Geometry: final body of the model. Coordinates: model frame, mm. Face numbers are marked on the shaded views. A direction names the side the tool comes from. Give positions to 0.01 mm unless a question says otherwise; leave off trailing zeros. Write each loop counter-clockwise with the first axis right and the second up, starting at its lowest first coordinate (ties: lowest second). Pieces come first, ordered by that corner, then holes. Notation, with made-up numbers: M -10.5,57.25 L 18.5,57.25 A26 ccw 18.5,80.25 Z; hole C 51.5,-28 d1. An arc over 180 degrees is marked long. One line per question, with ' | ' between items.
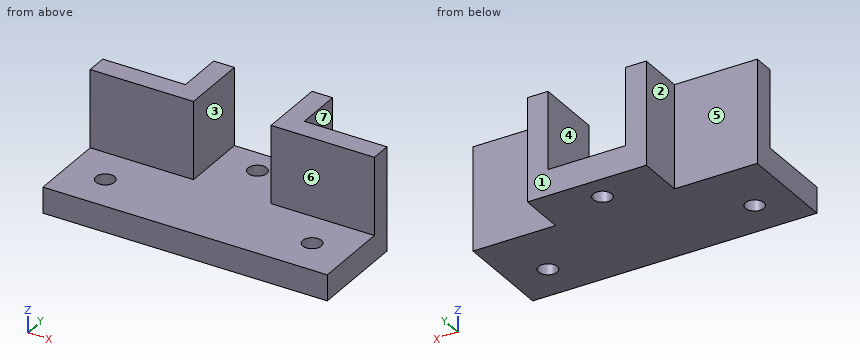
from build123d import *

# Parameters (mm, degrees)
BOSS_EXTRUDE1_DEPTH = 5
BOSS_EXTRUDE2_DEPTH = 20
SKETCH6_R           = 1.8
CUT_EXTRUDE3_DEPTH  = 6


with BuildPart() as part:
    # Sketch1 → Boss-Extrude1 (new body)
    with BuildSketch(Plane.XY):
        Polygon((14.31372549, 2.735294118), (34.31372549, 2.735294118), (34.31372549, -12.264705882), (-20.68627451, -12.264705882), (-20.68627451, 2.735294118), (-0.68627451, 2.735294118), (-0.68627451, 15.735294118), (14.31372549, 15.735294118), align=None)
    extrude(amount=BOSS_EXTRUDE1_DEPTH)

    # Sketch2 → Boss-Extrude2 (add)
    with BuildSketch(Plane(origin=(0, 0, 0), x_dir=(-1, 0, 0), z_dir=(0, 0, -1))):
        Polygon((0.68627451, 15.735294118), (4.68627451, 15.735294118), (4.68627451, 6.735294118), (6.079970528, 6.735294118), (20.68627451, 6.735294118), (20.68627451, 2.735294118), (0.68627451, 2.735294118), align=None)
    boss_extrude2 = extrude(amount=-BOSS_EXTRUDE2_DEPTH)

    # Mirror1: Boss-Extrude2 across plane
    add(boss_extrude2.mirror(Plane.ZY.offset(-6.81372549)))

    # Sketch6 → Cut-Extrude3 (cut, through all)
    with BuildSketch(Plane.XY.offset(5)):
        with Locations((6.81372549, 10.735294118)):
            Circle(SKETCH6_R)
        with Locations((-13.18627451, -4.764705882)):
            Circle(SKETCH6_R)
        with Locations((26.81372549, -4.764705882)):
            Circle(SKETCH6_R)
    extrude(amount=-CUT_EXTRUDE3_DEPTH, mode=Mode.SUBTRACT)


solid = part.part
(1) Cut plane A-A, the plane z = 6.75. Return loops of the section in (x, y).
Working result:
outline: M -20.69,2.74 L -0.69,2.74 L -0.69,15.74 L -4.69,15.74 L -4.69,6.74 L -20.69,6.74 Z; M 14.31,2.74 L 34.31,2.74 L 34.31,6.74 L 18.31,6.74 L 18.31,15.74 L 14.31,15.74 Z
(2) Material intervals for L1, parallel to X at y = 5, z = 14.5; L2, parallel to X at y = 14, z = 11.5; L3, parallel to X at y = -5, z = 1.75, sorted ascending. Write a range as [from, to].
Working result:
L1: x = [-20.69, -0.69], [14.31, 34.31] | L2: x = [-4.69, -0.69], [14.31, 18.31] | L3: x = [-20.69, -14.97], [-11.4, 25.03], [28.6, 34.31]
(3) Set-up query: the marked faces 4, 5, 6 and 7. Return all of +Z, -Z, +X, -X, +Y, -Y with unobstructed straight access to the full face (end or side cutting, diameter ignored); none if empty.
Working result:
face 4: +Z, +Y, -Y | face 5: +Z, -Z, -X, +Y | face 6: +Z, +X, -X, -Y | face 7: +Z, -Z, +X, +Y
(4) First-contact query: P1, Ø12, axis at x = 28, z = 11.5, coming from the -Y side; P2, Ø4, axis at x = 3.5, y = -6, coming from the +Z side; P3, Ø4.5, axis at y = 13, z = 10.5, coming from the +X side. Flat tips, straight axial feed; report the tip coordinate or a pass-through.
Working result:
P1: stops at y = 2.74 | P2: stops at z = 5 | P3: stops at x = 18.31
(5) Cut plane B-B, the plane y = 11.5. Return loops of the section in (x, z).
Working result:
outline: M -4.69,0 L 5.18,0 L 5.18,5 L -0.69,5 L -0.69,20 L -4.69,20 Z; M 8.44,0 L 18.31,0 L 18.31,20 L 14.31,20 L 14.31,5 L 8.44,5 Z
(6) Draft query along X for the marked faces 1, 2 and 3. Return one class per face: released by +X, released by -X, zero draft, split by the parting line, or undercut.
Working result:
face 1: zero draft | face 2: released by -X | face 3: undercut
(7) Cut plane C-C, the plane y = 4.75. Return loops of the section in (x, z).
Working result:
outline: M -20.69,0 L 34.31,0 L 34.31,20 L 14.31,20 L 14.31,5 L -0.69,5 L -0.69,20 L -20.69,20 Z
(8) Cut plane D-D, the plane x = -6.5. Return loops of the section in (y, z).
Working result:
outline: M -12.26,0 L 6.74,0 L 6.74,20 L 2.74,20 L 2.74,5 L -12.26,5 Z
